The model under review builds one solid part; all positions refer to its coordinate system, in mm. A direction names the side the tool comes from. Give positions to 0.01 mm unless a question says otherwise; leave off trailing zeros. Loops run counter-clockwise (first coordinate to the right, second up) from the corner with the lowest first, then second, coordinate; pieces in that order, holes last. Notation, with made-up numbers: M 45.5,-38 L 71.5,-38 A23 cw 71.5,-2 Z; hole C 12.25,87.5 d6. An arc over 180 degrees is marked long. One line per item, written item: value. Start each with the question number.
Q1. We need section C-C on x = 13. Write out the cut boundary in (y, z).
Q2. Mouldability with a two-part tool opening along Z and no side actions: class faces 1 (the face through (7, 20, 14)), 2 (the face through (13, 8, 29)), 3 (the face through (13, 1, 6)) as released by +Z, released by -Z, zero draft, split by the parting line, or undercut.
Q3. For pin 1 (3 mm diameter, centred on y = 15, z = 21, fed in from -X); pin 2 (1 mm diameter, centred on x = 5.5, z = 18, fed in from +Y); pin 3 (3 mm diameter, centred on y = 15, z = 20.5, fed in from +X), all flat-tipped, find the tip position at first contact; note any pin that passes through.
Q4. We need section A-A on y = 17.5. Write out the cut boundary in (x, z).
Q5. To check wall thickness, follow line 1 along X through (y, z) = (10.75, 19); line 2 along Z through (x, y) = (6.75, 2.25); line 3 along X through (y, z) = (1.5, 7.5). State the ranges of each line that lie inside material, in increasing order. Write a range as from..to.
Q6. We need section D-D on z = 25.25. Write out the cut boundary in (x, y), plus the area to 3 significant figures.
Q7. For faces 4 (the face through (6.2, 15, 15)), 5 (the face through (3, 20, 14)), 6 (the face through (13, 3, 15)), list the 3-axis set-ups (+Z, -Z, +X, -X, +Y, -Y) from which the entire face can be reached by the end or side of a thin tool; tool diameter is ignored.
```python
from build123d import *

# Parameters (mm, degrees)
F0_W     = 27
F0_H     = 20
F1_DEPTH = 29
F3_DEPTH = 29.001
F4_W     = 15
F4_H     = 17
F5_DEPTH = 3


with BuildPart() as f1:
    # F0 (on Top) → F1 (new body)
    with BuildSketch(Plane.XY):
        with Locations((13.5, 10)):
            Rectangle(F0_W, F0_H)
    extrude(amount=F1_DEPTH)

    # F2 (on face) → F3 (cut, through all)
    with BuildSketch(Plane.XY.offset(29)):
        Polygon((-5.87794, 25.212042), (-5.66129, 10), (2.2, 10), (2.2, 21), (4.2, 21), (4.2, 10), (6.2, 10), (6.2, 21), (8.2, 21), (8.2, 10), (10.2, 10), (10.2, 21), (12.2, 21), (12.2, 10), (14.2, 10), (14.2, 21), (16.2, 21), (16.2, 10), (18.2, 10), (18.2, 21), (20.2, 21), (20.2, 10), (22.2, 10), (22.2, 21), (24.2, 21), (24.2, 10), (26.2, 10), (30.417973, 10), (30.417973, 25.212042), align=None)
    extrude(amount=-F3_DEPTH, mode=Mode.SUBTRACT)

    # F4 (on face) → F5 (cut)
    with BuildSketch(Plane.XZ):
        with Locations((13.5, 14.5)):
            Rectangle(F4_W, F4_H)
    extrude(amount=-F5_DEPTH, mode=Mode.SUBTRACT)


solid = f1.part
```
Solved:
1. outline: M 0,0 L 10,0 L 10,29 L 0,29 L 0,23 L 3,23 L 3,6 L 0,6 Z
2. face 1: zero draft
2. face 2: released by +Z
2. face 3: undercut
3. pin 1: x = 2.2
3. pin 2: y = 10
3. pin 3: x = 24.2
4. outline: M 2.2,0 L 4.2,0 L 4.2,29 L 2.2,29 Z; M 6.2,0 L 8.2,0 L 8.2,29 L 6.2,29 Z; M 10.2,0 L 12.2,0 L 12.2,29 L 10.2,29 Z; M 14.2,0 L 16.2,0 L 16.2,29 L 14.2,29 Z; M 18.2,0 L 20.2,0 L 20.2,29 L 18.2,29 Z; M 22.2,0 L 24.2,0 L 24.2,29 L 22.2,29 Z
5. line 1: 2.2..4.2, 6.2..8.2, 10.2..12.2, 14.2..16.2, 18.2..20.2, 22.2..24.2
5. line 2: 0..6, 23..29
5. line 3: 0..6, 21..27
6. outline: M 0,0 L 27,0 L 27,10 L 24.2,10 L 24.2,20 L 22.2,20 L 22.2,10 L 20.2,10 L 20.2,20 L 18.2,20 L 18.2,10 L 16.2,10 L 16.2,20 L 14.2,20 L 14.2,10 L 12.2,10 L 12.2,20 L 10.2,20 L 10.2,10 L 8.2,10 L 8.2,20 L 6.2,20 L 6.2,10 L 4.2,10 L 4.2,20 L 2.2,20 L 2.2,10 L 0,10 Z
6. area: 390 mm2
7. face 4: +Z, -Z, +Y
7. face 5: +Z, -Z, +X, -X, +Y
7. face 6: -Y
